Build history of the part. All positions in model axes, mm. A direction names the side the tool comes from. Coordinates: 2 decimals unless noted, no trailing zeros. Order: outer loops, then holes, each group sorted by start corner. A loop starts at its lowest first (then second) coordinate and runs counter-clockwise, first axis right, second up. Notation, with made-up numbers: (-20, 55.25) - (-7, 55.25) arc R31 cw to (-7, 88.25) - close; hole circle Ø7 at (75, 34.5). An arc over 180 degrees is marked (long way). Write each question's results on one line, items separated by ' | '. Start each with the question number.
Autodesk Inventor part; units mm, degrees
ref_plane "YZ Plane" through (0, 0, 0) normal (1, 0, 0) x (0, 1, 0)
ref_plane "XZ Plane" through (0, 0, 0) normal (0, 1, 0) x (-1, 0, 0)
ref_plane "XY Plane" through (0, 0, 0) normal (0, 0, 1) x (1, 0, 0)
sketch "Sketch1" plane through (0, 0, 0) normal (1, 0, 0) x (0, 1, 0)
  line L0 (3.1935, -18.6702) -> (3.1935, -95.8243)
  arc A0 (3.1935, -95.8243) -> (7.9971, -98.5498) centre (6.3685, -95.8243) ccw
  arc A1 (7.9971, -98.5498) -> (58.1414, -63.3045) centre (-204.4103, 256.9406) ccw
  arc A2 (58.1414, -63.3045) -> (59.3034, -60.8492) centre (56.1284, -60.8492) ccw
  line L1 (59.3034, -60.8492) -> (59.3034, -56.7702)
  arc A3 (59.3034, -56.7702) -> (56.1284, -53.5952) centre (56.1284, -56.7702) ccw
  line L2 (56.1284, -53.5952) -> (34.9435, -53.5952)
  arc A4 (31.7685, -50.4202) -> (34.9435, -53.5952) centre (34.9435, -50.4202) ccw
  line L3 (31.7685, -50.4202) -> (31.7685, -21.8452)
  arc A5 (31.7685, -21.8452) -> (25.4185, -15.4952) centre (25.4185, -21.8452) ccw
  line L4 (25.4185, -15.4952) -> (6.3685, -15.4952)
  arc A6 (6.3685, -15.4952) -> (3.1935, -18.6702) centre (6.3685, -18.6702) ccw
  circle A7 centre (11.5501, -34.5452) radius 2.1844
  circle A8 centre (11.5501, -85.3452) radius 2.1844
  circle A9 centre (34.2518, -75.6387) radius 2.1844
  circle A10 centre (25.4185, -21.8452) radius 2.1844
  point P0 (0, 0)
  point P1 (25.4185, -15.4952)
  point P2 (3.1935, -18.6702)
  point P3 (7.9971, -98.5498)
  point P4 (58.1414, -63.3045)
  point P5 (34.9435, -53.5952)
sketch "Sketch2" plane through (1.5875, 0, 0) normal (1, 0, 0) x (0, 0, -1)
  line L0 (18.6702, 3.1935) -> (95.8243, 3.1935)
  line L1 (95.8243, 3.1935) -> (101.7995, 3.1935)
  arc A0 (63.3045, 58.1414) -> (60.8492, 59.3034) centre (60.8492, 56.1284) ccw
  line L2 (104.251, 8.3861) -> (63.3045, 58.1414)
  arc A1 (101.7995, 3.1935) -> (104.251, 8.3861) centre (101.7995, 6.3685) ccw
  arc A2 (98.5498, 7.9971) -> (63.3045, 58.1414) centre (-256.9406, -204.4103) ccw
  arc A3 (95.8243, 3.1935) -> (98.5498, 7.9971) centre (95.8243, 6.3685) ccw
  point P0 (0, 0)
  point P1 (108.5243, 3.1935)
  dimension "d1" = 12.7
  dimension "d2" = 3.175
extrude "Plate1" add sketch "Sketch1" along normal blind 1.5875
sheet face with bend "Face2" sketch "Sketch2" thickness 1.5875 toward (-1, 0, 0) bend radius 1.5875
bend "Bend1"
equation "\"d0\" = Thickness"
equation "\"d3\" = BendRadius"
equation "\"d4\" = BendReliefWidth"
equation "\"d6\" = MinimumRemnant"
equation "\"d5\" = BendReliefDepth"
equation "\"d7\" = TransitionRadius"
equation "\"BendRadius\" = Thickness"
equation "\"BendReliefWidth\" = Thickness"
equation "\"BendReliefDepth\" = 0.5 * Thickness"
equation "\"CornerReliefSize\" = 4 * Thickness"
equation "\"MinimumRemnant\" = 2 * Thickness"
equation "\"TransitionRadius\" = BendRadius"
equation "\"JacobiRadiusSize\" = BendRadius"
equation "\"GapSize\" = Thickness"
properties part number "sledsv3"
Item 1: Probe probe 1 along Z at (x, y) = (1.5, 12); probe 2 along Y at (x, z) = (0.7, -22); probe 3 along Z at (x, y) = (0.95, 6). List the from-to ranges inside material, lowest first.
Item 2: Which spindle directions (+Z, -Z, +X, -X, +Y, -Y) get a long thin tool onto all of the face, cutting with end or side? Do faces 1 (the flat face through (1, 46, -53.595)), 2 (the flat face through (1, 16, -15.495)). Say none if no direction does.
Item 3: Pull direction Y, two halves, no side cores. Call faces 3 (the cylindrical face through (0.8, 4.97, -104.65)), 4 (the flat face through (1, 3.194, -60)), 5 (the cylindrical face through (0.78, 12.72, -87.19)): released by +Y, released by -Y, zero draft, split by the parting line, or undercut.
Item 4: Slice it at A-A (z = -86.5). Write the cut outline in (x, y).
Item 5: Slice it at C-C (y = 19.5). Write the cut outline in (x, z), then the cut area to 3 significant figures.
Item 6: Slice it at B-B (x = 1.15). Count the separate pieces of the cut face and the enclosed holes in it, then the cut area to 3 significant figures.
Item 7: Slice it at D-D (z = -67.5). Write the cut outline in (x, y), then the cut area to 3 significant figures.
Resolved:
1) probe 1: -101.28 to -87.48, -83.21 to -36.68, -32.41 to -15.5 | probe 2: 3.19 to 23.24, 27.6 to 31.77 | probe 3: -104.95 to -15.52
2) face 1: +Z, +X, -X, +Y | face 2: +Z, +X, -X, +Y, -Y
3) face 3: split by the parting line | face 4: released by -Y | face 5: undercut
4) outline: (0, 3.19) - (1.59, 3.19) - (1.59, 9.7) - (0, 9.7) - close; (0, 13.4) - (1.59, 13.4) - (1.59, 29.96) - (0, 29.96) - close
5) outline: (0, -95.1) - (1.59, -95.1) - (1.59, -15.5) - (0, -15.5) - close | area: 126 mm^2
6) separate pieces: 1 | enclosed holes: 4 | area: 2,790 mm^2
7) outline: (0, 3.19) - (1.59, 3.19) - (1.59, 53.04) - (0, 53.04) - close | area: 79.1 mm^2
